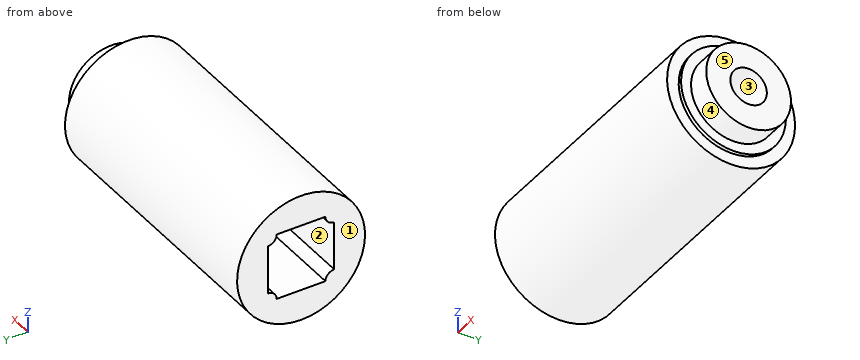
```python
from build123d import *

# Parameters (mm, degrees)
SKETCH1_R           = 54.345
BOSS_EXTRUDE1_DEPTH = 254
CUT_EXTRUDE1_DEPTH  = 100
SKETCH3_R           = 7
CUT_EXTRUDE2_DEPTH  = 139
SKETCH3_4_R         = 15.5
SKETCH3_4_R_2       = 7
CUT_EXTRUDE3_DEPTH  = 65
CUT_EXTRUDE4_START  = -23.5
SKETCH3_6_R         = 54.345
SKETCH3_6_R_2       = 44.5
CUT_EXTRUDE4_DEPTH  = 23.5
CUT_EXTRUDE5_START  = -20.3
SKETCH3_7_R         = 44.5
SKETCH3_7_R_2       = 36
CUT_EXTRUDE5_DEPTH  = 20.3
CHAMFER1_SIZE       = 10


with BuildPart() as part:
    # Sketch1 → Boss-Extrude1 (new body)
    with BuildSketch(Plane(origin=(0, 0, 0), x_dir=(0, 0, -1), z_dir=(1, 0, 0))):
        Circle(SKETCH1_R)
    extrude(amount=BOSS_EXTRUDE1_DEPTH)

    # Sketch2 → Cut-Extrude1 (cut)
    with BuildSketch(Plane(origin=(0, 0, 0), x_dir=(0, 0, -1), z_dir=(1, 0, 0))):
        with BuildLine():
            Line((20.694, 28.194), (-20.694, 28.194))
            ThreePointArc((-20.694, 28.194), (-22.890699141, 22.890699141), (-28.194, 20.694))
            Line((-28.194, 20.694), (-28.194, -20.694))
            ThreePointArc((-28.194, -20.694), (-22.890699141, -22.890699141), (-20.694, -28.194))
            Line((-20.694, -28.194), (20.694, -28.194))
            ThreePointArc((20.694, -28.194), (22.890699141, -22.890699141), (28.194, -20.694))
            Line((28.194, -20.694), (28.194, 20.694))
            ThreePointArc((28.194, 20.694), (22.890699141, 22.890699141), (20.694, 28.194))
        make_face()
    extrude(amount=CUT_EXTRUDE1_DEPTH, mode=Mode.SUBTRACT)

    # Sketch3 → Cut-Extrude2 (cut)
    with BuildSketch(Plane(origin=(254, 0, 0), x_dir=(0, 0, -1), z_dir=(1, 0, 0))):
        Circle(SKETCH3_R)
    extrude(amount=-CUT_EXTRUDE2_DEPTH, mode=Mode.SUBTRACT)

    # Sketch3<4> → Cut-Extrude3 (cut)
    with BuildSketch(Plane(origin=(254, 0, 0), x_dir=(0, 0, -1), z_dir=(1, 0, 0))):
        Circle(SKETCH3_4_R)
        Circle(SKETCH3_4_R_2, mode=Mode.SUBTRACT)
    extrude(amount=-CUT_EXTRUDE3_DEPTH, mode=Mode.SUBTRACT)

    # Sketch3<6> → Cut-Extrude4 (cut)
    with BuildSketch(Plane(origin=(254, 0, 0), x_dir=(0, 0, -1), z_dir=(1, 0, 0)).offset(CUT_EXTRUDE4_START)):
        Circle(SKETCH3_6_R)
        Circle(SKETCH3_6_R_2, mode=Mode.SUBTRACT)
    extrude(amount=CUT_EXTRUDE4_DEPTH, mode=Mode.SUBTRACT)

    # Sketch3<7> → Cut-Extrude5 (cut)
    with BuildSketch(Plane(origin=(254, 0, 0), x_dir=(0, 0, -1), z_dir=(1, 0, 0)).offset(CUT_EXTRUDE5_START)):
        Circle(SKETCH3_7_R)
        Circle(SKETCH3_7_R_2, mode=Mode.SUBTRACT)
    extrude(amount=CUT_EXTRUDE5_DEPTH, mode=Mode.SUBTRACT)

    # Chamfer1
    # the kernel refuses this chamfer: 10 mm, written as the material it adds along each edge
    with BuildSketch(Plane(origin=(189, 0, 0), x_dir=(0, 0, -1), z_dir=(0, -1, 0))) as chamfer1_piece_1_section:
        Polygon((15.5, CHAMFER1_SIZE), (15.5 - CHAMFER1_SIZE, 0), (15.5, 0), align=None)
    chamfer1_piece_1 = revolve(axis=Axis((189, 0, 0), (1, 0, 0)), mode=Mode.PRIVATE)
    chamfer1_piece_1 = chamfer1_piece_1 - Plane(origin=(194.777828899, 0, 0), x_dir=(0, 0, -1), z_dir=(1, 0, 0)) * Cylinder(7, 62, mode=Mode.PRIVATE)
    add(chamfer1_piece_1)


solid = part.part
```
Here's how the part is built. I have some questions about the finished solid (model axes, mm). Face numbers are marked on the shaded views. A direction names the side the tool comes from. Coordinates: 2 decimals unless noted, no trailing zeros. Order: outer loops, then holes, each group sorted by start corner. A loop starts at its lowest first (then second) coordinate and runs counter-clockwise, first axis right, second up. Notation, with made-up numbers: M 80,37 L 98,37 A30 cw 98,70 Z; hole C 88.5,12.5 d2. An arc over 180 degrees is marked long. Answer as a JSON object with one key per item and string values. Group by question number.
(1) Suppose I cut it at A-A, the plane x = 36. Please give me the cut outline in (y, z) (3 decimals).
(2) If we mould it in two halves opening along Y, with no side actions, what happens to the marked faces 3, 4 and 5? For each: released by +Y, released by -Y, zero draft, split by the parting line, or undercut.
(3) Which directions (+Z, -Z, +X, -X, +Y, -Y) give clear straight access to the entire face, cutting with the end or side of a thin tool? Please do the marked faces 1 and 2.
(4) Suppose I cut it at D-D, the plane x = 106. Please give me the cut outline in (y, z) (3 decimals), then the cut area to 3 significant figures.
(5) Suppose I cut it at B-B, the plane y = 0. Please give me the cut outline in (x, z) (3 decimals).
(6) For pin 1 (6 mm diameter, centred on x = 219.5, y = -1, fed in from -Z) (3 decimals); pin 2 (17 mm diameter, centred on y = 0, z = -8, fed in from -X); pin 3 (11 mm diameter, centred on y = -2.5, z = -3, fed in from +X); pin 4 (1.5 mm diameter, centred on x = 76, y = 30, fed in from -Z), each with a flat end and sliding along its axis, tell me the tip position at first contact or that it passes through.
(7) I need wall thicknesses on probe 1 along Y at (x, z) = (228, 0) (3 decimals); probe 2 along Y at (x, z) = (13, 0.5); probe 3 along X at (y, z) = (-16, -20.5). Which ranges of each line are inside material? Lowest first, please.
Values found:
{
 "1": {"outline": "C 0,0 d108.69; hole M -28.194,-20.694 A7.5 cw -20.694,-28.194 L 20.694,-28.194 A7.5 cw 28.194,-20.694 L 28.194,20.694 A7.5 cw 20.694,28.194 L -20.694,28.194 A7.5 cw -28.194,20.694 Z"},
 "2": {"face 3": "undercut", "face 4": "split by the parting line", "face 5": "zero draft"},
 "3": {"face 1": "+Z, -Z, -X, +Y, -Y", "face 2": "-X"},
 "4": {"outline": "C 0,0 d108.69", "area": "9,280 mm^2"},
 "5": {"outline": "M 0,-54.345 L 230.5,-54.345 L 230.5,-44.5 L 233.7,-44.5 L 233.7,-36 L 254,-36 L 254,-15.5 L 199,-15.5 L 190.5,-7 L 115,-7 L 115,7 L 190.5,7 L 199,15.5 L 254,15.5 L 254,36 L 233.7,36 L 233.7,44.5 L 230.5,44.5 L 230.5,54.345 L 0,54.345 L 0,28.194 L 100,28.194 L 100,-28.194 L 0,-28.194 Z"},
 "6": {"pin 1": "stops at z = -54.345", "pin 2": "stops at x = 100", "pin 3": "stops at x = 192.91", "pin 4": "stops at z = -45.8"},
 "7": {"probe 1": "y = -54.345 to -15.5, 15.5 to 54.345", "probe 2": "y = -54.34 to -28.19, 28.19 to 54.34", "probe 3": "x = 100 to 254"}
}
